Can you work these out from the model? Positions are in its coordinate system, mm. A direction names the side the tool comes from. Give positions to 0.01 mm unless a question says otherwise; leave off trailing zeros. Order: outer loops, then holes, each group sorted by start corner. A loop starts at its lowest first (then second) coordinate and runs counter-clockwise, first axis right, second up. Notation, with made-up numbers: (-15, 81) -> (33, 81) arc R7 ccw to (33, 90) -> close; hole circle Ø5 at (-27.5, 40.25). An arc over 180 degrees is marked (long way). Answer as CSV lines item,"result".
```python
from build123d import *

# Parameters (mm, degrees)
SKETCH_1_W      = 32
SKETCH_1_H      = 55
EXTRUDE_1_DEPTH = 12
EXTRUDE_2_DEPTH = 12
SKETCH_2_R      = 2.5
EXTRUDE_3_DEPTH = 12
SKETCH_3_R      = 1.75
EXTRUDE_4_DEPTH = 12
FILLET_1_R      = 3


with BuildPart() as part:
    # Sketch 1 → Extrude 1 (new body)
    with BuildSketch(Plane(origin=(0, 0, 0), x_dir=(1, 0, 0), z_dir=(0, 1, 0))):
        Rectangle(SKETCH_1_W, SKETCH_1_H)
    extrude(amount=EXTRUDE_1_DEPTH)

    # Sketch 1_3 → Extrude 2 (add)
    with BuildSketch(Plane(origin=(0, 0, 0), x_dir=(1, 0, 0), z_dir=(0, 1, 0))):
        Polygon((0, -27.5), (-16, -27.5), (-12.5, -47.5), (0, -47.5), align=None)
        Polygon((12.5, -47.5), (16, -27.5), (0, -27.5), (0, -47.5), align=None)
    extrude(amount=EXTRUDE_2_DEPTH)

    # Sketch 2 → Extrude 3 (add)
    with BuildSketch(Plane.XY.offset(47.5)):
        with Locations(Location((6, 6, 0), (0, 0, 180))):
            Circle(SKETCH_2_R)
        with Locations(Location((-6, 6, 0), (0, 0, 180))):
            Circle(SKETCH_2_R)
    extrude(amount=EXTRUDE_3_DEPTH)

    # Sketch 3 → Extrude 4 (add)
    with BuildSketch(Plane(origin=(0, 0, -27.5), x_dir=(-1, 0, 0), z_dir=(0, 0, -1))):
        with BuildLine():
            ThreePointArc((1.75, 6), (1.237436867, 7.237436867), (0, 7.75))
            Line((0, 7.75), (0, 4.25))
            ThreePointArc((0, 4.25), (1.237436867, 4.762563133), (1.75, 6))
        make_face()
        with BuildLine():
            Line((0, 4.25), (0, 7.75))
            ThreePointArc((0, 7.75), (-1.75, 6), (0, 4.25))
        make_face()
        with Locations((8, 6)):
            Circle(SKETCH_3_R)
        with Locations((-8, 6)):
            Circle(SKETCH_3_R)
    extrude(amount=EXTRUDE_4_DEPTH)

    # Fillet 1
    fillet_1_edges = [part.edges().sort_by_distance(p)[0] for p in [
        (0, 0, 47.5),
        (-12.5, 6, 47.5),
        (12.5, 6, 47.5),
        (0, 12, 47.5),
        (0, 12, -27.5),
        (0, 0, -27.5),
        (-16, 6, -27.5),
        (16, 6, -27.5),
    ]]
    fillet(fillet_1_edges, radius=FILLET_1_R)


solid = part.part
```
Item 1: Imagine slicing it at A-A, the plane x = -12. Please give me the cut outline in (y, z).
Numbers:
outline,"(0, -24.5) arc R3 ccw to (3, -27.5) -> (9, -27.5) arc R3 ccw to (12, -24.5) -> (12, 44.5) arc R3 ccw to (11.02, 46.72) -> (0.98, 46.72) arc R3 ccw to (0, 44.5) -> close"
Item 2: For faces 1 (the cylindrical face through (-8.81, 4.45, -33.42)), 2 (the flat face through (16, 6, 2)), 3 (the cylindrical face through (3.615, 5.249, 53.416)), which set-ups out of +Z, -Z, +X, -X, +Y, -Y let a thin tool reach every point of the face, with its end or its side?
Numbers:
face 1,"-Z"
face 2,"+Z, -Z, +X, +Y, -Y"
face 3,"+Z"
Item 3: For pin 1 (3 mm diameter, centred on x = -4, y = 6, fed in from -Z); pin 2 (1.5 mm diameter, centred on x = 12, y = 3, fed in from +Z); pin 3 (6 mm diameter, centred on x = -1.5, y = 10, fed in from +Z), each with a flat end and sliding along its axis, tell me the tip position at first contact or that it passes through.
Numbers:
pin 1,"stops at z = -27.5"
pin 2,"stops at z = 47.22"
pin 3,"stops at z = 47.5"
Item 4: We'd pull the mould along X, two halves only. Please class faces 4 (the cylindrical face through (15.438, 6.084, -26.248)), 5 (the flat face through (0, 8, -27.5)), 6 (the flat face through (8, 6, -39.5)): released by +X, released by -X, zero draft, split by the parting line, or undercut.
Numbers:
face 4,"released by +X"
face 5,"undercut"
face 6,"zero draft"
Item 5: Please list where these lines run through material, in increasing order: line 1 along Z through (x, y) = (4, 4); line 2 along X through (y, z) = (5, 38); line 3 along X through (y, z) = (7.5, 54.5).
Numbers:
line 1,"z = -27.5 to 47.5"
line 2,"x = -14.16 to 14.16"
line 3,"x = -8 to -4, 4 to 8"
Item 6: Imagine slicing it at B-B, the plane y = 1.5. Please give me the cut outline in (x, z), then the cut area to 3 significant figures.
Numbers:
outline,"(-16, -24.5) arc R3 ccw to (-14.5, -27.1) -> (14.5, -27.1) arc R3 ccw to (16, -24.5) -> (16, 27.5) -> (12.93, 45.02) arc R3 ccw to (11.48, 47.1) -> (-11.48, 47.1) arc R3 ccw to (-12.93, 45.02) -> (-16, 27.5) -> close"
area,"2,300 mm²"
Item 7: Imagine slicing it at C-C, the plane z = 32.5. Please give me the cut outline in (x, y) (3 decimals), then the cut area to 3 significant figures.
Numbers:
outline,"(-15.125, 0) -> (15.125, 0) -> (15.125, 12) -> (-15.125, 12) -> close"
area,"363 mm²"
